Autodesk Inventor part; units mm, degrees
ref_plane "YZ Plane" through (0, 0, 0) normal (1, 0, 0) x (0, 1, 0)
ref_plane "XZ Plane" through (0, 0, 0) normal (0, 1, 0) x (-1, 0, 0)
ref_plane "XY Plane" through (0, 0, 0) normal (0, 0, 1) x (1, 0, 0)
sketch "Sketch1" plane through (0, 0, 0) normal (0, 0, 1) x (1, 0, 0)
  circle A0 centre (0, 0) radius 30
  dimension "d0" = 60
extrude "Extrusion1" add sketch "Sketch1" along normal blind 3
sketch "Sketch2" plane through (0, 0, 3) normal (0, 0, 1) x (1, 0, 0)
  circle A0 centre (0, 0) radius 30
  circle A1 centre (30, 30) radius 25
  dimension "d6" = 50
  dimension "d7" = 30
  dimension "d8" = 30
extrude "Extrusion2" cut sketch "Sketch2" against normal through all contours A1 A0 | A0 A1 picked at (18.8229, 17.5315) picked at (30.2504, 29.5845)
pattern_circular "Circular Pattern1" count 5 over 360 about axis through (0, 0, -10) along (0, 0, 1) of "Extrusion2"
sketch "Sketch3" plane through (0, 0, 3) normal (0, 0, 1) x (1, 0, 0)
  point P0 (0, 0)
  point P1 (0, 0)
hole "Hole1" at (0, 0, 3) direction (0, 0, -1) diameter 5.5 end through all
properties part number "Timing_Star"
Input: part model. Units: mm. Frame: model coordinates. Coordinates: 2 decimals unless noted, no trailing zeros. Order: outer loops, then holes, each group sorted by start corner. A loop starts at its lowest first (then second) coordinate and runs counter-clockwise, first axis right, second up. Notation, with made-up numbers: M 46,24.25 L 72,24.25 A12 ccw 72,32.25 Z; hole C 7.5,9.5 d4. An arc over 180 degrees is marked long. Answer as CSV lines item,"result".
1. Section D-D (y = -7). Return the cut outline in (x, z), then the cut area to 3 significant figures.
Reported:
outline,"M -16.91,0 L 16.02,0 L 16.02,3 L -16.91,3 Z"
area,"98.8 mm2"
2. First-contact query: P1, Ø1.5, axis at x = -14.5, z = 0.5, coming from the -Y side; P2, Ø1, axis at y = -7.5, z = 1.5, coming from the -X side. Flat tips, straight axial feed; report the tip coordinate or a pass-through.
Reported:
P1,"y = -18.43"
P2,"x = -16.94"
3. Pull-direction query (X, two-part tool) for faces 1 (the cylindrical face through (-17.17, -2.99, 1.52)), 2 (the cylindrical face through (12.133, 12.514, 1.521)), 3 (the flat face through (1, -4, 3)), 4 (the cylindrical face through (2.685, 0.596, 1.479)); classes: released by +X, released by -X, zero draft, split by the parting line, or undercut.
Reported:
face 1,"released by -X"
face 2,"released by +X"
face 3,"zero draft"
face 4,"undercut"
4. Section B-B (x = 0). Return the cut outline in (y, z), then the cut area to 3 significant figures.
Reported:
outline,"M -17.8,0 L -2.75,0 L -2.75,3 L -17.8,3 Z; M 2.75,0 L 21.86,0 L 21.86,3 L 2.75,3 Z"
area,"102 mm2"
5. Material intervals for line 1 (Y direction, x = 0, z = 2); line 2 (X direction, y = 2.5, z = 1.6), sorted ascending. Write a range as from..to.
Reported:
line 1,"-17.8..-2.75, 2.75..21.86"
line 2,"-18.63..-1.15, 1.15..25.5"
6. Section A-A (z = 2.4). Return the cut outline in (x, y), then the cut area to 3 significant figures.
Reported:
outline,"M -26.87,13.34 A25 cw -21.43,-20.99 A30 ccw -20.99,-21.43 A25 cw 13.34,-26.87 A30 ccw 13.9,-26.59 A25 cw 29.68,4.38 A30 ccw 29.58,5 A25 cw 5,29.58 A30 ccw 4.38,29.68 A25 cw -26.59,13.9 A30 ccw Z; hole C 0,0 d5.5"
area,"1,310 mm2"
